```python
from build123d import *

# Parameters (mm, degrees)
SKETCH1_W               = 25
SKETCH1_H               = 67
BOSS_EXTRUDE1_DEPTH     = 1
SKETCH2_W               = 1
SKETCH2_H               = 67
BOSS_EXTRUDE2_DEPTH     = 24
SKETCH3_W               = 1
SKETCH3_H               = 25
BOSS_EXTRUDE3_DEPTH     = 10
SKETCH4_W               = 1
SKETCH4_H               = 25
BOSS_EXTRUDE4_DEPTH     = 10
SKETCH5_R               = 5
CUT_EXTRUDE1_DEPTH      = 2
SKETCH10_R              = 1.5
CUT_EXTRUDE3_DEPTH      = 68
CUT_EXTRUDE4_DEPTH      = 11
CUT_EXTRUDE4_DEPTH_BACK = 36
SKETCH9_R               = 5
CUT_EXTRUDE2_DEPTH      = 36


with BuildPart() as part:
    # Sketch1 → Boss-Extrude1 (new body)
    with BuildSketch(Plane(origin=(0, 0, 0), x_dir=(1, 0, 0), z_dir=(0, 1, 0))):
        Rectangle(SKETCH1_W, SKETCH1_H)
    extrude(amount=BOSS_EXTRUDE1_DEPTH)

    # Sketch2 → Boss-Extrude2 (add)
    with BuildSketch(Plane(origin=(0, 1, 0), x_dir=(1, 0, 0), z_dir=(0, 1, 0))):
        with Locations((12, 0)):
            Rectangle(SKETCH2_W, SKETCH2_H)
        with Locations((-12, 0)):
            Rectangle(SKETCH2_W, SKETCH2_H)
    extrude(amount=BOSS_EXTRUDE2_DEPTH)

    # Sketch3 → Boss-Extrude3 (add)
    with BuildSketch(Plane(origin=(12.5, 0, 0), x_dir=(0, 0, -1), z_dir=(1, 0, 0))):
        with Locations((-33, 12.5)):
            Rectangle(SKETCH3_W, SKETCH3_H)
        with Locations((33, 12.5)):
            Rectangle(SKETCH3_W, SKETCH3_H)
    extrude(amount=BOSS_EXTRUDE3_DEPTH)

    # Sketch4 → Boss-Extrude4 (add)
    with BuildSketch(Plane.ZY.offset(12.5)):
        with Locations((-33, 12.5)):
            Rectangle(SKETCH4_W, SKETCH4_H)
        with Locations((33, 12.5)):
            Rectangle(SKETCH4_W, SKETCH4_H)
    extrude(amount=BOSS_EXTRUDE4_DEPTH)

    # Sketch5 → Cut-Extrude1 (cut, through all)
    with BuildSketch(Plane(origin=(0, 1, 0), x_dir=(1, 0, 0), z_dir=(0, 1, 0))):
        with Locations((0, -11.5)):
            Circle(SKETCH5_R)
        with Locations((0, 15.5)):
            Circle(SKETCH5_R)
    extrude(amount=-CUT_EXTRUDE1_DEPTH, mode=Mode.SUBTRACT)

    # Sketch10 → Cut-Extrude3 (cut, through all)
    with BuildSketch(Plane.XY.offset(33.5)):
        with Locations((17, 20)):
            Circle(SKETCH10_R)
        with Locations((17, 5)):
            Circle(SKETCH10_R)
        with Locations((-17, 20)):
            Circle(SKETCH10_R)
        with Locations((-17, 5)):
            Circle(SKETCH10_R)
    extrude(amount=-CUT_EXTRUDE3_DEPTH, mode=Mode.SUBTRACT)

    # Sketch11 → Cut-Extrude4 (cut, two sides)
    with BuildSketch(Plane(origin=(12.5, 0, 0), x_dir=(0, 0, -1), z_dir=(1, 0, 0))) as cut_extrude4_sk:
        Polygon((0, 25), (-23.5, 25), (-18.5, 20), (0, 20), align=None)
        Polygon((23.5, 25), (0, 25), (0, 20), (18.5, 20), align=None)
    extrude(amount=CUT_EXTRUDE4_DEPTH, mode=Mode.SUBTRACT)
    extrude(cut_extrude4_sk.sketch, amount=-CUT_EXTRUDE4_DEPTH_BACK, mode=Mode.SUBTRACT)

    # Sketch9 → Cut-Extrude2 (cut, through all)
    with BuildSketch(Plane(origin=(12.5, 0, 0), x_dir=(0, 0, -1), z_dir=(1, 0, 0))):
        with Locations((-11.5, 10)):
            Circle(SKETCH9_R)
        with Locations((15.5, 10)):
            Circle(SKETCH9_R)
    extrude(amount=-CUT_EXTRUDE2_DEPTH, mode=Mode.SUBTRACT)


solid = part.part
```
Design review of the part built by this model. Coordinates are the model's own, in mm. A direction names the side the tool comes from. Round coordinates to 2 decimals unless told otherwise and drop trailing zeros. Write each loop counter-clockwise with the first axis right and the second up, starting at its lowest first coordinate (ties: lowest second). Pieces come first, ordered by that corner, then holes. Notation, with made-up numbers: (26.25, -14.5) -> (51.25, -14.5) arc R22 ccw to (51.25, 22.5) -> close; hole circle Ø5 at (-35.5, -12). An arc over 180 degrees is marked (long way). Answer in a Markdown table with one row per item.
Q1. Take a section at B-B, the plane x = 0. State the section outline as (y, z) points.
The answers:
| item | result |
|---|---|
| outline | (0, -33.5) -> (1, -33.5) -> (1, -20.5) -> (0, -20.5) -> close; (0, -10.5) -> (1, -10.5) -> (1, 6.5) -> (0, 6.5) -> close; (0, 16.5) -> (1, 16.5) -> (1, 33.5) -> (0, 33.5) -> close |
Q2. Draft analysis for pull direction X (two halves, no side actions). For faces 1 (the face through (-15, 25, -33)), 2 (the face through (11.5, 13, 0)), 3 (the face through (-18.11, 21.01, 33.01)), state which applies: +X half, -X half, draft (parallel to the pull), parting line (faces both ways), or undercut.
The answers:
| item | result |
|---|---|
| face 1 | draft |
| face 2 | undercut |
| face 3 | undercut |
Q3. Take a section at D-D, the plane z = 1.5. State the section outline as (x, y) points, then the cut area to 3 significant figures.
The answers:
| item | result |
|---|---|
| outline | (-12.5, 0) -> (12.5, 0) -> (12.5, 20) -> (11.5, 20) -> (11.5, 1) -> (-11.5, 1) -> (-11.5, 20) -> (-12.5, 20) -> close |
| area | 63.0 mm² |
Q4. Clearance check with flat-ended pins moving along their axes: pin 1 Ø7.5 at (y, z) = (16.5, -10.5) entering from -X; pin 2 Ø4 at (x, y) = (17, 20) entering from -Z; pin 3 Ø3 at (y, z) = (6.5, -0.5) entering from +X; pin 4 Ø0.8 at (x, z) = (-12, -7.5) entering from +Y. State where each tip first meets the part, or that it passes through.
The answers:
| item | result |
|---|---|
| pin 1 | x = -12.5 |
| pin 2 | z = -33.5 |
| pin 3 | x = 12.5 |
| pin 4 | y = 20 |
Q5. For faces 4 (the face through (17, 12, 32.5)), 5 (the face through (-12, 22.5, -21)), 6 (the face through (-17, 12, -32.5)), list the 3-axis set-ups (+Z, -Z, +X, -X, +Y, -Y) from which the entire face can be reached by the end or side of a thin tool; tool diameter is ignored.
The answers:
| item | result |
|---|---|
| face 4 | +X, +Y, -Y |
| face 5 | +X, -X, +Y |
| face 6 | -X, +Y, -Y |
Q6. Take a section at A-A, the plane z = 11.5. State the section outline as (x, y) points, then the cut area to 3 significant figures.
The answers:
| item | result |
|---|---|
| outline | (-12.5, 0) -> (-5, 0) -> (-5, 1) -> (-11.5, 1) -> (-11.5, 5) -> (-12.5, 5) -> close; (-12.5, 15) -> (-11.5, 15) -> (-11.5, 20) -> (-12.5, 20) -> close; (5, 0) -> (12.5, 0) -> (12.5, 5) -> (11.5, 5) -> (11.5, 1) -> (5, 1) -> close; (11.5, 15) -> (12.5, 15) -> (12.5, 20) -> (11.5, 20) -> close |
| area | 33.0 mm² |
Q7. Take a section at C-C, the plane x = 17. State the section outline as (y, z) points, then the cut area to 3 significant figures.
The answers:
| item | result |
|---|---|
| outline | (0, -33.5) -> (3.5, -33.5) -> (3.5, -32.5) -> (0, -32.5) -> close; (0, 32.5) -> (3.5, 32.5) -> (3.5, 33.5) -> (0, 33.5) -> close; (6.5, -33.5) -> (18.5, -33.5) -> (18.5, -32.5) -> (6.5, -32.5) -> close; (6.5, 32.5) -> (18.5, 32.5) -> (18.5, 33.5) -> (6.5, 33.5) -> close; (21.5, -33.5) -> (25, -33.5) -> (25, -32.5) -> (21.5, -32.5) -> close; (21.5, 32.5) -> (25, 32.5) -> (25, 33.5) -> (21.5, 33.5) -> close |
| area | 38.0 mm² |
Q8. To check wall thickness, follow L1, parallel to Y at x = -17, z = -33.3; L2, parallel to Y at x = 12, z = 11.5; L3, parallel to Z at x = 16.5, y = 12.5. State the ranges of each line that lie inside material, in increasing order. Write a range as [from, to].
The answers:
| item | result |
|---|---|
| L1 | [0, 3.5], [6.5, 18.5], [21.5, 25] |
| L2 | [0, 5], [15, 20] |
| L3 | [-33.5, -32.5], [32.5, 33.5] |
